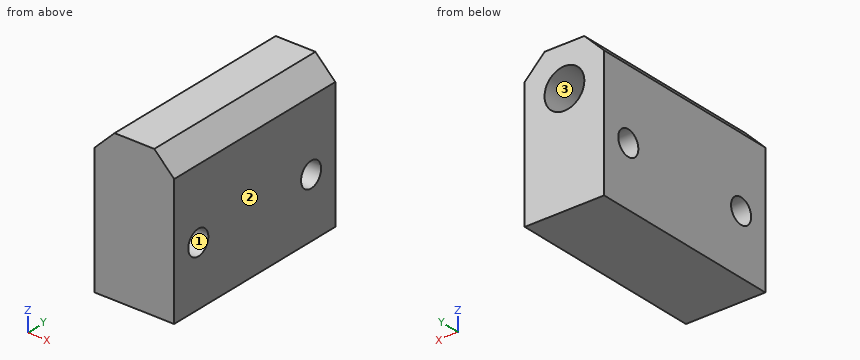
```python
from build123d import *

# Parameters (mm, degrees)
SKETCH1_W                    = 16
SKETCH1_H                    = 30
BOSS_EXTRUDE1_DEPTH          = 40
O_0_316_DIAMETER_HOLE1_D     = 8.0264
O_0_316_DIAMETER_HOLE1_DEPTH = 15
O_0_316_DIAMETER_HOLE1_TIP   = 2.411373836
F_10_CLEARANCE_HOLE1_D       = 4.9784
CHAMFER1_SIZE                = 4


with BuildPart() as part:
    # Sketch1 → Boss-Extrude1 (new body)
    with BuildSketch(Plane(origin=(0, 0, 0), x_dir=(1, 0, 0), z_dir=(0, 1, 0))):
        with Locations((0, 7)):
            Rectangle(SKETCH1_W, SKETCH1_H)
    extrude(amount=BOSS_EXTRUDE1_DEPTH)

    # O (0.316) Diameter Hole1
    with Locations(Plane(origin=(0, 40, 0), x_dir=(1, 0, 0), z_dir=(0, 1, 0))):
        with Locations((0, 0)):
            Hole(O_0_316_DIAMETER_HOLE1_D / 2, depth=O_0_316_DIAMETER_HOLE1_DEPTH)
            with Locations((0, 0, -(O_0_316_DIAMETER_HOLE1_DEPTH + O_0_316_DIAMETER_HOLE1_TIP / 2))):  # 118° drill point
                Cone(0, O_0_316_DIAMETER_HOLE1_D / 2, O_0_316_DIAMETER_HOLE1_TIP, mode=Mode.SUBTRACT)

    # #10 Clearance Hole1 (through all)
    with Locations(Plane.ZY.offset(8)):
        with Locations((-10, 34), (-10, 6)):
            Hole(F_10_CLEARANCE_HOLE1_D / 2)

    # Chamfer1
    chamfer1_edges = [part.edges().sort_by_distance(p)[0] for p in [
        (8, 20, 8),
        (-8, 20, 8),
    ]]
    chamfer(chamfer1_edges, length=CHAMFER1_SIZE)


solid = part.part
```
Geometry check sheet. Reference: the model listing, model coordinates, mm. Face numbers are marked on the shaded views. Coordinates: 2 decimals unless noted, no trailing zeros. Write each loop counter-clockwise with the first axis right and the second up, starting at its lowest first coordinate (ties: lowest second). Pieces come first, ordered by that corner, then holes. Notation, with made-up numbers: M -18,28 L 34,28 A13 ccw 34,47 Z; hole C -33,21.5 d10. An arc over 180 degrees is marked long. Use one line per item in the form item = value. Start each with the question number.
1) Section check C-C on x = -6.5. Enter the section's corners in (y, z).
2) Section check D-D on z = -10. Enter the section's corners in (x, y).
3) Section check A-A on y = 34. Enter the section's corners in (x, z).
4) Release check for a two-part mould opening along X. For the marked faces 1, 2 and 3 record: pulls with the +X half, pulls with the -X half, needs draft (parallel to the pull), parting line crosses it, or undercut.
5) Section check B-B on y = 6. Enter the section's corners in (x, z), and give its area (3 significant figures).
6) Thickness scan on probe 1 along Y at (x, z) = (-2.5, -10); probe 2 along Z at (x, y) = (0, 29); probe 3 along Z at (x, y) = (0, 36). Record the ranges inside material, lowest first. Write a range as from..to.
Responses:
q1.outline = M 0,-22 L 40,-22 L 40,5.5 L 0,5.5 Z; hole C 6,-10 d4.98; hole C 34,-10 d4.98
q2.outline = M -8,0 L 8,0 L 8,3.51 L -8,3.51 Z; M -8,8.49 L 8,8.49 L 8,31.51 L -8,31.51 Z; M -8,36.49 L 8,36.49 L 8,40 L -8,40 Z
q3.outline = M -8,-22 L 8,-22 L 8,-12.49 L -8,-12.49 Z; M -8,-7.51 L 8,-7.51 L 8,4 L 4,8 L -4,8 L -8,4 Z; hole C 0,0 d8.03
q4.face_1 = needs draft
q4.face_2 = pulls with the +X half
q4.face_3 = undercut
q5.outline = M -8,-22 L 8,-22 L 8,-12.49 L -8,-12.49 Z; M -8,-7.51 L 8,-7.51 L 8,4 L 4,8 L -4,8 L -8,4 Z
q5.area = 384 mm2
q6.probe_1 = 0..3.51, 8.49..31.51, 36.49..40
q6.probe_2 = -22..-4.01, 4.01..8
q6.probe_3 = -22..-11.48, -8.52..-4.01, 4.01..8
